```python
from build123d import *

# Parameters (mm, degrees)
F1_DEPTH = 152.4
F2_W     = 127
F2_H     = 152.4
F3_DEPTH = 152.4
F5_DEPTH = 76.2
F7_DEPTH = 76.2


with BuildPart() as f1:
    # F0 (on Front) → F1 (new body)
    with BuildSketch(Plane.XZ):
        with BuildLine():
            Line((-330.2, 495.3), (-330.2, -495.3))
            Line((-330.2, -495.3), (-203.2, -495.3))
            Line((-203.2, -495.3), (-203.2, 63.5))
            ThreePointArc((-203.2, 63.5), (0, 266.7), (203.2, 63.5))
            Line((203.2, 63.5), (203.2, -495.3))
            Line((203.2, -495.3), (330.2, -495.3))
            Line((330.2, -495.3), (330.2, 495.3))
            Line((330.2, 495.3), (-330.2, 495.3))
        make_face()
    extrude(amount=F1_DEPTH)

    # F2 (on face) → F3 (join)
    with BuildSketch(Plane(origin=(0, 0, 0), x_dir=(-1, 0, 0), z_dir=(0, 1, 0))):
        with Locations((-266.7, -419.1)):
            Rectangle(F2_W, F2_H)
        with Locations((266.7, -419.1)):
            Rectangle(F2_W, F2_H)
    extrude(amount=F3_DEPTH)

    # F4 (on face) → F5 (cut)
    with BuildSketch(Plane(origin=(-330.2, 0, 0), x_dir=(0, -1, 0), z_dir=(-1, 0, 0))):
        with BuildLine():
            ThreePointArc((76.2, 298.45), (107.630896, 311.469104), (120.65, 342.9))
            Line((120.65, 342.9), (76.2, 342.9))
            Line((76.2, 342.9), (76.2, 298.45))
        make_face()
        with BuildLine():
            Line((76.2, 342.9), (120.65, 342.9))
            ThreePointArc((120.65, 342.9), (44.769104, 374.330896), (76.2, 298.45))
            Line((76.2, 298.45), (76.2, 342.9))
        make_face()
        with BuildLine():
            ThreePointArc((124.425977, -317.5), (110.300915, -283.399085), (76.2, -269.274023))
            ThreePointArc((76.2, -269.274023), (42.099085, -351.600915), (124.425977, -317.5))
        make_face()
        with BuildLine():
            ThreePointArc((120.65, 12.7), (107.630896, 44.130896), (76.2, 57.15))
            Line((76.2, 57.15), (76.2, 12.7))
            Line((76.2, 12.7), (76.2, -31.75))
            ThreePointArc((76.2, -31.75), (107.630896, -18.730896), (120.65, 12.7))
        make_face()
        with BuildLine():
            Line((76.2, 12.7), (76.2, 57.15))
            ThreePointArc((76.2, 57.15), (31.75, 12.7), (76.2, -31.75))
            Line((76.2, -31.75), (76.2, 12.7))
        make_face()
    extrude(amount=-F5_DEPTH, mode=Mode.SUBTRACT)

    # F6 (on face) → F7 (cut)
    with BuildSketch(Plane.YZ.offset(330.2)):
        with BuildLine():
            ThreePointArc((-76.2, 298.45), (-44.769104, 311.469104), (-31.75, 342.9))
            ThreePointArc((-31.75, 342.9), (-107.630896, 374.330896), (-76.2, 298.45))
        make_face()
        with BuildLine():
            ThreePointArc((-31.75, -317.5), (-44.769104, -286.069104), (-76.2, -273.05))
            ThreePointArc((-76.2, -273.05), (-107.630896, -348.930896), (-31.75, -317.5))
        make_face()
        with BuildLine():
            ThreePointArc((-31.75, 12.7), (-44.769104, 44.130896), (-76.2, 57.15))
            Line((-76.2, 57.15), (-76.2, 12.7))
            Line((-76.2, 12.7), (-76.2, -31.75))
            ThreePointArc((-76.2, -31.75), (-44.769104, -18.730896), (-31.75, 12.7))
        make_face()
        with BuildLine():
            Line((-76.2, 12.7), (-76.2, 57.15))
            ThreePointArc((-76.2, 57.15), (-120.65, 12.7), (-76.2, -31.75))
            Line((-76.2, -31.75), (-76.2, 12.7))
        make_face()
    extrude(amount=-F7_DEPTH, mode=Mode.SUBTRACT)


solid = f1.part
```
Can you work these out from the model? Positions are in its coordinate system, mm. A direction names the side the tool comes from. Round coordinates to 2 decimals unless told otherwise and drop trailing zeros. Loops run counter-clockwise (first coordinate to the right, second up) from the corner with the lowest first, then second, coordinate; pieces in that order, holes last. Notation, with made-up numbers: (-27, 9.25) -> (-17, 9.25) arc R23 cw to (-17, 28.25) -> close; hole circle Ø2 at (-10.5, 73). An arc over 180 degrees is marked (long way). One line per item, written item: value. Start each with the question number.
1. For faces 1 (the flat face through (-254, -76, 13)), 2 (the flat face through (-266, 75, -342.9)), 3 (the flat face through (-203.2, -32, -282)), 4 (the flat face through (254, -77, 344)), which set-ups out of +Z, -Z, +X, -X, +Y, -Y let a thin tool reach every point of the face, with its end or its side?
2. If we section it at C-C, the plane x = -276: Write out the boundary of the cut face in (y, z).
3. If we section it at A-A, the plane z = -240: Write out the boundary of the cut face in (x, y).
4. If I drill on probe 1 along Z at (x, y) = (312, -76.2); probe 2 along Z at (x, y) = (-283, -76); probe 3 along Y at (x, z) = (273, -317), over which ranges is the centre line in solid material (lowest first)?
5. If we section it at B-B, the plane y = 17.5: Write out the boundary of the cut face in (x, z).
6. If we mould it in two halves opening along Z, with no side actions, what happens to faces 5 (the flat face through (-254, -76, -317)), 6 (the flat face through (268, 75, -342.9)), 7 (the flat face through (-330.2, -66, -103))? For each: pulls with the +Z half, pulls with the -Z half, needs draft (parallel to the pull), parting line crosses it, or undercut.
Calculated:
1. face 1: -X
1. face 2: +Z, +X, -X, +Y
1. face 3: -Z, +Y, -Y
1. face 4: +X
2. outline: (-152.4, -495.3) -> (152.4, -495.3) -> (152.4, -342.9) -> (0, -342.9) -> (0, 495.3) -> (-152.4, 495.3) -> close; hole (-124.43, -317.5) arc R48.23 ccw (long way) to (-76.2, -269.27) arc R48.23 ccw to start; hole (-120.65, 12.7) arc R44.45 ccw to (-76.2, -31.75) arc R44.45 ccw to (-76.2, 57.15) arc R44.45 ccw to start; hole (-120.65, 342.9) arc R44.45 ccw to (-76.2, 298.45) arc R44.45 ccw (long way) to start
3. outline: (-330.2, -152.4) -> (-203.2, -152.4) -> (-203.2, 0) -> (-330.2, 0) -> close; (203.2, -152.4) -> (330.2, -152.4) -> (330.2, 0) -> (203.2, 0) -> close
4. probe 1: z = -495.3 to -361.95, -273.05 to -31.75, 57.15 to 298.45, 387.35 to 495.3
4. probe 2: z = -495.3 to -365.73, -269.27 to -31.75, 57.15 to 298.45, 387.35 to 495.3
4. probe 3: y = -152.4 to -120.65, -31.75 to 0
5. outline: (-330.2, -495.3) -> (-203.2, -495.3) -> (-203.2, -342.9) -> (-330.2, -342.9) -> close; (203.2, -495.3) -> (330.2, -495.3) -> (330.2, -342.9) -> (203.2, -342.9) -> close
6. face 5: undercut
6. face 6: pulls with the +Z half
6. face 7: needs draft
